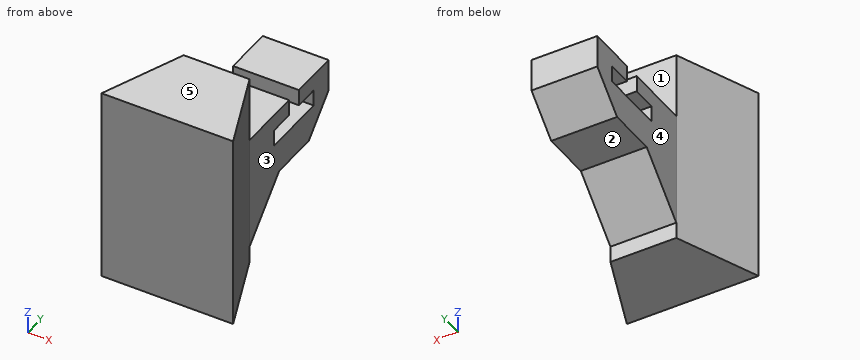
```python
from build123d import *

# Parameters (mm, degrees)
BOSS_EXTRUDE1_DEPTH = 12
SKETCH2_W           = 4
SKETCH2_H           = 4
BOSS_EXTRUDE2_DEPTH = 8
CHAMFER1_SIZE       = 3
CUT_EXTRUDE1_DEPTH  = 18
CHAMFER2_SIZE       = 2


with BuildPart() as part:
    # Sketch1 → Boss-Extrude1 (new body)
    with BuildSketch(Plane.XY):
        Polygon((-3.130434783, -2.608695652), (4.869565217, -2.608695652), (2.869565217, 2.391304348), (-1.130434783, 2.391304348), align=None)
    extrude(amount=BOSS_EXTRUDE1_DEPTH)

    # Sketch2 → Boss-Extrude2 (add)
    with BuildSketch(Plane(origin=(0, 2.391304348, 0), x_dir=(1, 0, 0), z_dir=(0, 1, 0))):
        with Locations((0.869565217, -6)):
            Rectangle(SKETCH2_W, SKETCH2_H)
    extrude(amount=BOSS_EXTRUDE2_DEPTH)

    # Chamfer1
    chamfer1_edges = [part.edges().sort_by_distance(p)[0] for p in [
        (0.869565217, 2.391304348, 4),
    ]]
    chamfer(chamfer1_edges, length=CHAMFER1_SIZE)

    # Sketch3 → Cut-Extrude1 (cut)
    with BuildSketch(Plane(origin=(2.869565217, 0, 0), x_dir=(0, 0, -1), z_dir=(1, 0, 0))):
        Polygon((-7, 8.891304348), (-6, 8.891304348), (-6, 4.891304348), (-7, 4.891304348), (-7, 6.391304348), (-8, 6.391304348), (-8, 7.391304348), (-7, 7.391304348), align=None)
    extrude(amount=-CUT_EXTRUDE1_DEPTH, mode=Mode.SUBTRACT)

    # Chamfer2
    chamfer2_edges = [part.edges().sort_by_distance(p)[0] for p in [
        (0.869565217, 10.391304348, 4),
    ]]
    chamfer(chamfer2_edges, length=CHAMFER2_SIZE)


solid = part.part
```
The model under review builds one solid part; all positions refer to its coordinate system, in mm. Face numbers are marked on the shaded views. A direction names the side the tool comes from. Round coordinates to 2 decimals unless told otherwise and drop trailing zeros. Write each loop counter-clockwise with the first axis right and the second up, starting at its lowest first coordinate (ties: lowest second). Pieces come first, ordered by that corner, then holes. Notation, with made-up numbers: (-13.75, 87.25) - (33.25, 87.25) arc R23 ccw to (33.25, 121.25) - close; hole circle Ø7 at (65.25, 86). An arc over 180 degrees is marked (long way). Answer as CSV lines item,"result". Start each with the question number.
(1) We need section B-B on x = 2. State the section outline as (y, z) points.
(2) To check wall thickness, follow line 1 (Z direction, x = -0.25, y = 6); line 2 (Y direction, x = 2.75, z = 8.5); line 3 (Y direction, x = 2.75, z = 7.75). State the ranges of each line that lie inside material, in increasing order.
(3) We need section D-D on z = 9.75. State the section outline as (x, y) points.
(4) For pin 1 Ø1 at (y, z) = (4.5, 2.5) entering from +X; pin 2 Ø5 at (y, z) = (4.5, 7.5) entering from -X; pin 3 Ø1.6 at (x, y) = (0, 8) entering from -Z, all flat-tipped, find the tip position at first contact; note any pin that passes through.
(5) For the marked faces 1, 2, 3, 4 and 5, list the 3-axis set-ups (+Z, -Z, +X, -X, +Y, -Y) from which the entire face can be reached by the end or side of a thin tool; tool diameter is ignored.
(6) We need section C-C on z = 3.5. State the section outline as (x, y) points.
(7) We need section A-A on y = 8. State the section outline as (x, z) points.
Worked answers:
1,outline,"(-2.61, 0) - (2.39, 0) - (2.39, 1) - (5.39, 4) - (8.39, 4) - (10.39, 6) - (10.39, 8) - (7.39, 8) - (7.39, 7) - (8.89, 7) - (8.89, 6) - (4.89, 6) - (4.89, 7) - (6.39, 7) - (6.39, 8) - (2.39, 8) - (2.39, 12) - (-2.61, 12) - close"
2,line 1,"4 to 6, 7 to 8"
2,line 2,"-2.61 to 2.39"
2,line 3,"-2.61 to 6.39, 7.39 to 10.39"
3,outline,"(-3.13, -2.61) - (4.87, -2.61) - (2.87, 2.39) - (-1.13, 2.39) - close"
4,pin 1,"x = 2.87"
4,pin 2,"x = -1.29"
4,pin 3,"z = 4"
5,face 1,"+Z, +X, -X, +Y"
5,face 2,"-Z, +X, -X, +Y"
5,face 3,"+Z, -Z, +X, +Y"
5,face 4,"+Z, -Z, -X, +Y"
5,face 5,"+Z, +X, -X, +Y, -Y"
6,outline,"(-3.13, -2.61) - (4.87, -2.61) - (2.87, 2.39) - (2.87, 4.89) - (-1.13, 4.89) - (-1.13, 2.39) - close"
7,outline,"(-1.13, 4) - (2.87, 4) - (2.87, 6) - (-1.13, 6) - close; (-1.13, 7) - (2.87, 7) - (2.87, 8) - (-1.13, 8) - close"
